The drawing under review shows one solid part. Ordinate dimensions are in mm from its lowest x, y, z. Give positions to 0.01 mm unless a question says otherwise; leave off trailing zeros. Loops run counter-clockwise (first coordinate to the right, second up) from the corner with the lowest first, then second, coordinate; pieces in that order, holes last. Notation, with made-up numbers: M 77.5,12 L 134.5,12 A14 ccw 134.5,38 Z; hole C 60,5 d6. An arc over 180 degrees is marked long. Put each result on its own line as item: value. Start each with the question number.
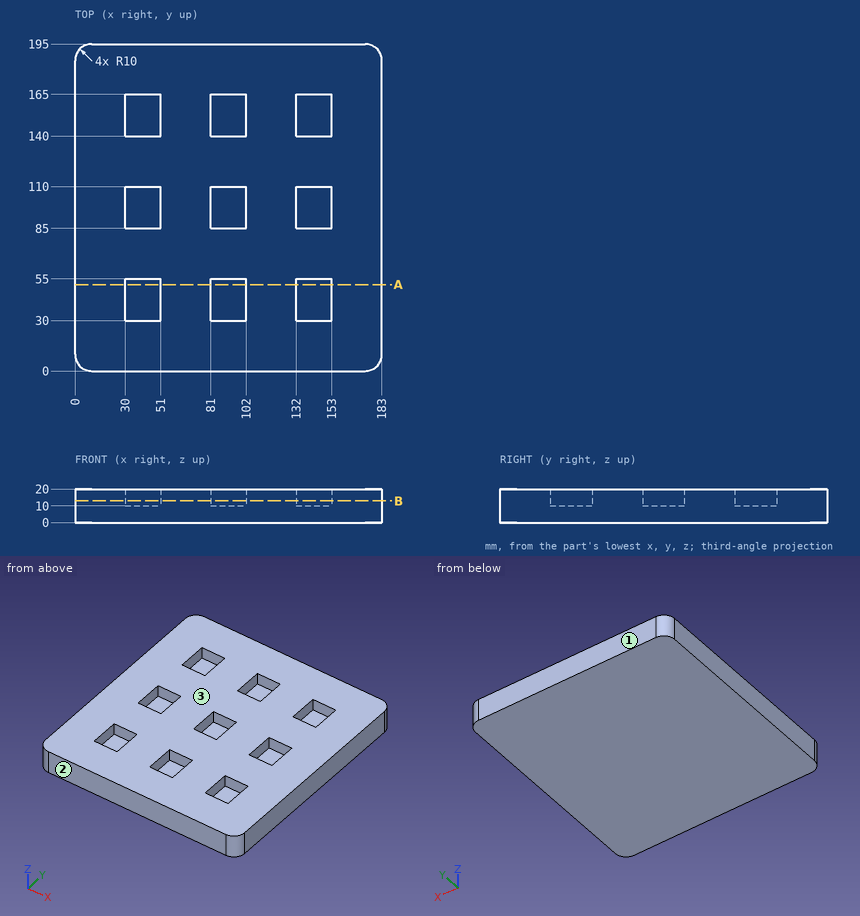
(1) Insertion check: pin 1 (5 mm diameter, centred on x = 108.5, y = 32, fed in from -Z). The pin has a flat end and moves straight along its axis. Give the tip position at first contact, or say it passes through.
(2) We need section A-A, the plane y = 51.5. Write out the cut boundary in (x, z).
(3) Draft analysis for pull direction Y (two halves, no side actions). For the marked faces 1, 2 and 3, state which applies: +Y half, -Y half, draft (parallel to the pull), parting line (faces both ways), or undercut.
(4) To check wall thickness, follow L1, parallel to Y at x = 133, z = 13; L2, parallel to X at y = 44, z = 13; L3, parallel to Z at x = 89, y = 101. State the ranges of each line that lie inside material, in increasing order. Write a range as [from, to].
(5) We need section B-B, the plane z = 13. State how many separate pieces and enclosed holes the cut face has, plus the area to 3 significant figures.
Check sheet entries:
1. pin 1: stops at z = 0
2. outline: M 0,0 L 183,0 L 183,20 L 153,20 L 153,10 L 132,10 L 132,20 L 102,20 L 102,10 L 81,10 L 81,20 L 51,20 L 51,10 L 30,10 L 30,20 L 0,20 Z
3. face 1: +Y half
3. face 2: -Y half
3. face 3: draft
4. L1: y = [0, 30], [55, 85], [110, 140], [165, 195]
4. L2: x = [0, 30], [51, 81], [102, 132], [153, 183]
4. L3: z = [0, 10]
5. separate pieces: 1
5. enclosed holes: 9
5. area: 30,900 mm²
